```python
from build123d import *

# Parameters (mm, degrees)
SALIENTE_EXTRUIR1_DEPTH      = 30
SALIENTE_EXTRUIR1_DEPTH_BACK = 30
CROQUIS1_W                   = 110
CROQUIS1_H                   = 20
CORTAR_EXTRUIR1_REACH        = 67.765
CROQUIS2_R                   = 20
CROQUIS3_R                   = 5.5
CORTAR_EXTRUIR2_DEPTH        = 7
CORTAR_EXTRUIR3_REACH        = 65.984
CROQUIS4_R                   = 3.25
CORTAR_EXTRUIR4_REACH        = 67.765
CROQUIS5_R                   = 5.5


with BuildPart() as part:
    # Croquis1 → Saliente-Extruir1 (new, two sides: drawn at the far end of the back side and taken through both)
    with BuildSketch(Plane(origin=(0, 0, 0), x_dir=(0, 0, -1), z_dir=(1, 0, 0)).offset(-SALIENTE_EXTRUIR1_DEPTH_BACK)):
        with Locations((0, -10)):
            Rectangle(CROQUIS1_W, CROQUIS1_H)
    extrude(amount=SALIENTE_EXTRUIR1_DEPTH + SALIENTE_EXTRUIR1_DEPTH_BACK)

    # Croquis2 → Cortar-Extruir1 (cut, up to next)
    with BuildSketch(Plane(origin=(0, 0, 0), x_dir=(1, 0, 0), z_dir=(0, 1, 0)), mode=Mode.PRIVATE) as cortar_extruir1_sk1:
        with Locations(Location((0, 0, 0), (0, 0, 270))):
            Circle(CROQUIS2_R)
    cortar_extruir1_tool1 = extrude(cortar_extruir1_sk1.sketch, amount=-CORTAR_EXTRUIR1_REACH, mode=Mode.PRIVATE) & part.part
    add(cortar_extruir1_tool1.solids().sort_by_distance((0, 0, 0))[0], mode=Mode.SUBTRACT)

    # Croquis3 → Cortar-Extruir2 (cut)
    with BuildSketch(Plane(origin=(0, 0, 0), x_dir=(1, 0, 0), z_dir=(0, 1, 0))):
        with Locations(Location((-21, 21, 0), (0, 0, 270))):
            Circle(CROQUIS3_R)
        with Locations(Location((21, 21, 0), (0, 0, 270))):
            Circle(CROQUIS3_R)
        with Locations(Location((21, -21, 0), (0, 0, 270))):
            Circle(CROQUIS3_R)
        with Locations(Location((-21, -21, 0), (0, 0, 270))):
            Circle(CROQUIS3_R)
    extrude(amount=-CORTAR_EXTRUIR2_DEPTH, mode=Mode.SUBTRACT)

    # Croquis4 → Cortar-Extruir3 (cut, up to next)
    with BuildSketch(Plane(origin=(0, -7, 0), x_dir=(1, 0, 0), z_dir=(0, 1, 0)), mode=Mode.PRIVATE) as cortar_extruir3_sk1:
        with Locations(Location((-21, 21, 0), (0, 0, 270))):
            Circle(CROQUIS4_R)
    cortar_extruir3_tool1 = extrude(cortar_extruir3_sk1.sketch, amount=-CORTAR_EXTRUIR3_REACH, mode=Mode.PRIVATE) & part.part
    # Croquis4 → Cortar-Extruir3 (cut, up to next)
    with BuildSketch(Plane(origin=(0, -7, 0), x_dir=(1, 0, 0), z_dir=(0, 1, 0)), mode=Mode.PRIVATE) as cortar_extruir3_sk2:
        with Locations(Location((21, 21, 0), (0, 0, 270))):
            Circle(CROQUIS4_R)
    cortar_extruir3_tool2 = extrude(cortar_extruir3_sk2.sketch, amount=-CORTAR_EXTRUIR3_REACH, mode=Mode.PRIVATE) & part.part
    # Croquis4 → Cortar-Extruir3 (cut, up to next)
    with BuildSketch(Plane(origin=(0, -7, 0), x_dir=(1, 0, 0), z_dir=(0, 1, 0)), mode=Mode.PRIVATE) as cortar_extruir3_sk3:
        with Locations(Location((21, -21, 0), (0, 0, 270))):
            Circle(CROQUIS4_R)
    cortar_extruir3_tool3 = extrude(cortar_extruir3_sk3.sketch, amount=-CORTAR_EXTRUIR3_REACH, mode=Mode.PRIVATE) & part.part
    # Croquis4 → Cortar-Extruir3 (cut, up to next)
    with BuildSketch(Plane(origin=(0, -7, 0), x_dir=(1, 0, 0), z_dir=(0, 1, 0)), mode=Mode.PRIVATE) as cortar_extruir3_sk4:
        with Locations(Location((-21, -21, 0), (0, 0, 270))):
            Circle(CROQUIS4_R)
    cortar_extruir3_tool4 = extrude(cortar_extruir3_sk4.sketch, amount=-CORTAR_EXTRUIR3_REACH, mode=Mode.PRIVATE) & part.part
    add(cortar_extruir3_tool1.solids().sort_by_distance((-21, -7, -21))[0], mode=Mode.SUBTRACT)
    add(cortar_extruir3_tool2.solids().sort_by_distance((21, -7, -21))[0], mode=Mode.SUBTRACT)
    add(cortar_extruir3_tool3.solids().sort_by_distance((21, -7, 21))[0], mode=Mode.SUBTRACT)
    add(cortar_extruir3_tool4.solids().sort_by_distance((-21, -7, 21))[0], mode=Mode.SUBTRACT)

    # Croquis5 → Cortar-Extruir4 (cut, up to next)
    with BuildSketch(Plane(origin=(0, 0, 0), x_dir=(1, 0, 0), z_dir=(0, 1, 0)), mode=Mode.PRIVATE) as cortar_extruir4_sk1:
        with Locations(Location((-20, 45, 0), (0, 0, 270))):
            Circle(CROQUIS5_R)
    cortar_extruir4_tool1 = extrude(cortar_extruir4_sk1.sketch, amount=-CORTAR_EXTRUIR4_REACH, mode=Mode.PRIVATE) & part.part
    # Croquis5 → Cortar-Extruir4 (cut, up to next)
    with BuildSketch(Plane(origin=(0, 0, 0), x_dir=(1, 0, 0), z_dir=(0, 1, 0)), mode=Mode.PRIVATE) as cortar_extruir4_sk2:
        with Locations(Location((20, 45, 0), (0, 0, 270))):
            Circle(CROQUIS5_R)
    cortar_extruir4_tool2 = extrude(cortar_extruir4_sk2.sketch, amount=-CORTAR_EXTRUIR4_REACH, mode=Mode.PRIVATE) & part.part
    # Croquis5 → Cortar-Extruir4 (cut, up to next)
    with BuildSketch(Plane(origin=(0, 0, 0), x_dir=(1, 0, 0), z_dir=(0, 1, 0)), mode=Mode.PRIVATE) as cortar_extruir4_sk3:
        with Locations(Location((20, -45, 0), (0, 0, 270))):
            Circle(CROQUIS5_R)
    cortar_extruir4_tool3 = extrude(cortar_extruir4_sk3.sketch, amount=-CORTAR_EXTRUIR4_REACH, mode=Mode.PRIVATE) & part.part
    # Croquis5 → Cortar-Extruir4 (cut, up to next)
    with BuildSketch(Plane(origin=(0, 0, 0), x_dir=(1, 0, 0), z_dir=(0, 1, 0)), mode=Mode.PRIVATE) as cortar_extruir4_sk4:
        with Locations(Location((-20, -45, 0), (0, 0, 270))):
            Circle(CROQUIS5_R)
    cortar_extruir4_tool4 = extrude(cortar_extruir4_sk4.sketch, amount=-CORTAR_EXTRUIR4_REACH, mode=Mode.PRIVATE) & part.part
    add(cortar_extruir4_tool1.solids().sort_by_distance((-20, 0, -45))[0], mode=Mode.SUBTRACT)
    add(cortar_extruir4_tool2.solids().sort_by_distance((20, 0, -45))[0], mode=Mode.SUBTRACT)
    add(cortar_extruir4_tool3.solids().sort_by_distance((20, 0, 45))[0], mode=Mode.SUBTRACT)
    add(cortar_extruir4_tool4.solids().sort_by_distance((-20, 0, 45))[0], mode=Mode.SUBTRACT)


solid = part.part
```
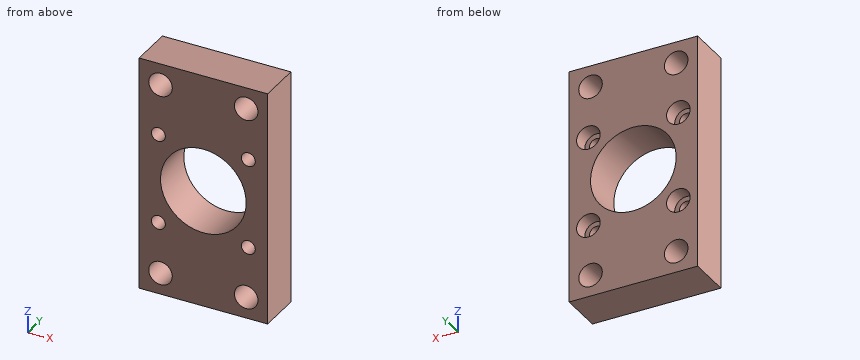
CAD build for the part. Positions are in the model's coordinates, mm. Coordinates: 2 decimals unless noted, no trailing zeros. Loops run counter-clockwise (first coordinate to the right, second up) from the corner with the lowest first, then second, coordinate; pieces in that order, holes last. Notation, with made-up numbers: (3, 75.25) - (45, 75.25) arc R29 cw to (45, 107.25) - close; hole circle Ø7 at (77.25, 74.25). An arc over 180 degrees is marked (long way). Use CSV: the item, a comma, the result in double quotes. Start each with the question number.
Q1. Cut at B-B, the plane y = -2.75. State how many separate pieces and enclosed holes the cut face has, then the cut area to 3 significant figures.
Q2. Cut at C-C, the plane x = -4.5. List the corners of the cut face in (y, z).
Q3. Cut at A-A, the plane z = 45. List the corners of the cut face in (x, y), then the cut area to 3 significant figures.
Q4. Drop flat-ended pins along their axis: P1, Ø5, axis at x = 20.5, z = 43, coming from the -Y side; P2, Ø3.5, axis at x = -22, z = 23.5, coming from the +Y side. Give the stop position or say it passes through.
Q5. Cut at D-D, the plane z = 0. List the corners of the cut face in (x, y), then the cut area to 3 significant figures.
Q6. Probe probe 1 along X at (y, z) = (-7.25, 45); probe 2 along X at (y, z) = (-15, -21); probe 3 along Z at (x, y) = (-18, -1.25). List the from-to ranges inside material, lowest first. Write a range as from..to.
Here are the results:
1,separate pieces,"1"
1,enclosed holes,"9"
1,area,"4,580 mm2"
2,outline,"(-20, -55) - (0, -55) - (0, -19.49) - (-20, -19.49) - close; (-20, 19.49) - (0, 19.49) - (0, 55) - (-20, 55) - close"
3,outline,"(-30, -20) - (-25.5, -20) - (-25.5, 0) - (-30, 0) - close; (-14.5, -20) - (14.5, -20) - (14.5, 0) - (-14.5, 0) - close; (25.5, -20) - (30, -20) - (30, 0) - (25.5, 0) - close"
3,area,"760 mm2"
4,P1,"through"
4,P2,"y = -7"
5,outline,"(-30, -20) - (-20, -20) - (-20, 0) - (-30, 0) - close; (20, -20) - (30, -20) - (30, 0) - (20, 0) - close"
5,area,"400 mm2"
6,probe 1,"-30..-25.5, -14.5..14.5, 25.5..30"
6,probe 2,"-30..-24.25, -17.75..17.75, 24.25..30"
6,probe 3,"-55..-50.12, -39.88..-25.61, -16.39..-8.72, 8.72..16.39, 25.61..39.88, 50.12..55"
